Source: three-view drawing plus pictorial views. Frame: mm from the lowest corner of the part. Give positions to 0.01 mm unless a question says otherwise; leave off trailing zeros. Write each loop counter-clockwise with the first axis right and the second up, starting at its lowest first coordinate (ties: lowest second). Pieces come first, ordered by that corner, then holes.
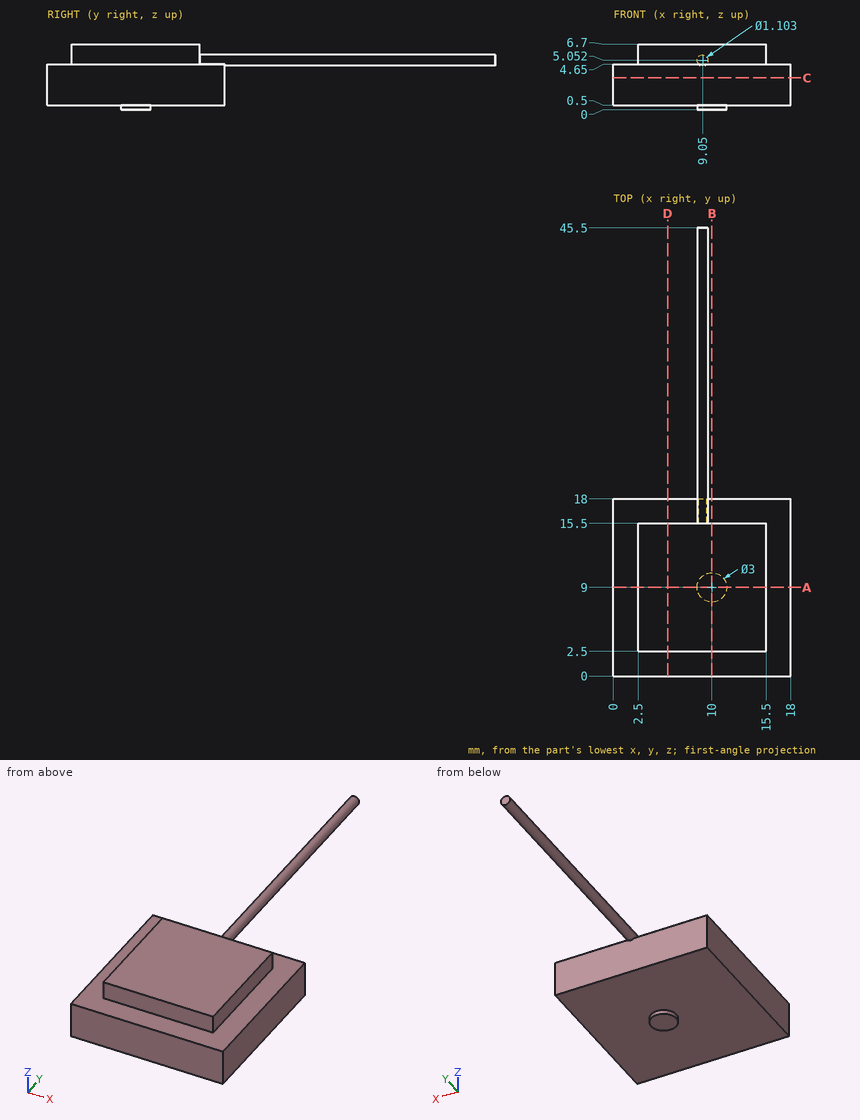
Q1. Section D-D on x = 5.5. Output: boundary loops of the cut face in (y, z), plus the area to 3 significant figures.
Filled sheet:
outline: (0, 0.5) - (18, 0.5) - (18, 4.65) - (15.5, 4.65) - (15.5, 6.7) - (2.5, 6.7) - (2.5, 4.65) - (0, 4.65) - close
area: 101 mm2
Q2. Section B-B on x = 10. Output: boundary loops of the cut face in (y, z).
Filled sheet:
outline: (0, 0.5) - (7.5, 0.5) - (7.5, 0) - (10.5, 0) - (10.5, 0.5) - (18, 0.5) - (18, 4.65) - (15.5, 4.65) - (15.5, 6.7) - (2.5, 6.7) - (2.5, 4.65) - (0, 4.65) - close
Q3. Pin query (flat end, axial travel): P1, Ø1, axis at x = 8.5, y = 33.5, coming from the -Z side; P2, Ø1.6, axis at y = 10, z = 5.5, coming from the -X side; P3, Ø1.2, axis at x = 9.5, z = 3.5, coming from the +Y side. Return the tip coordinate at first contact, or that it passes through.
Filled sheet:
P1: stops at z = 4.5
P2: stops at x = 2.5
P3: stops at y = 18
Q4. Section C-C on z = 3.25. Output: boundary loops of the cut face in (x, y).
Filled sheet:
outline: (0, 0) - (18, 0) - (18, 18) - (0, 18) - close
Q5. Ray query, line 1 along Z through (x, y) = (5.25, 13); line 2 along Y through (x, z) = (7, 2); line 3 along Z through (x, y) = (4.5, 17.5). Return the intervals inside material, ascending.
Filled sheet:
line 1: z = 0.5 to 6.7
line 2: y = 0 to 18
line 3: z = 0.5 to 4.65
Q6. Section A-A on y = 9. Output: boundary loops of the cut face in (x, z).
Filled sheet:
outline: (0, 0.5) - (8.5, 0.5) - (8.5, 0) - (11.5, 0) - (11.5, 0.5) - (18, 0.5) - (18, 4.65) - (15.5, 4.65) - (15.5, 6.7) - (2.5, 6.7) - (2.5, 4.65) - (0, 4.65) - close
